Check sheet for the drawn part. Datum: minimum x, y, z corner. Units: mm. Coordinates: 2 decimals unless noted, no trailing zeros. Loops run counter-clockwise (first coordinate to the right, second up) from the corner with the lowest first, then second, coordinate; pieces in that order, holes last.
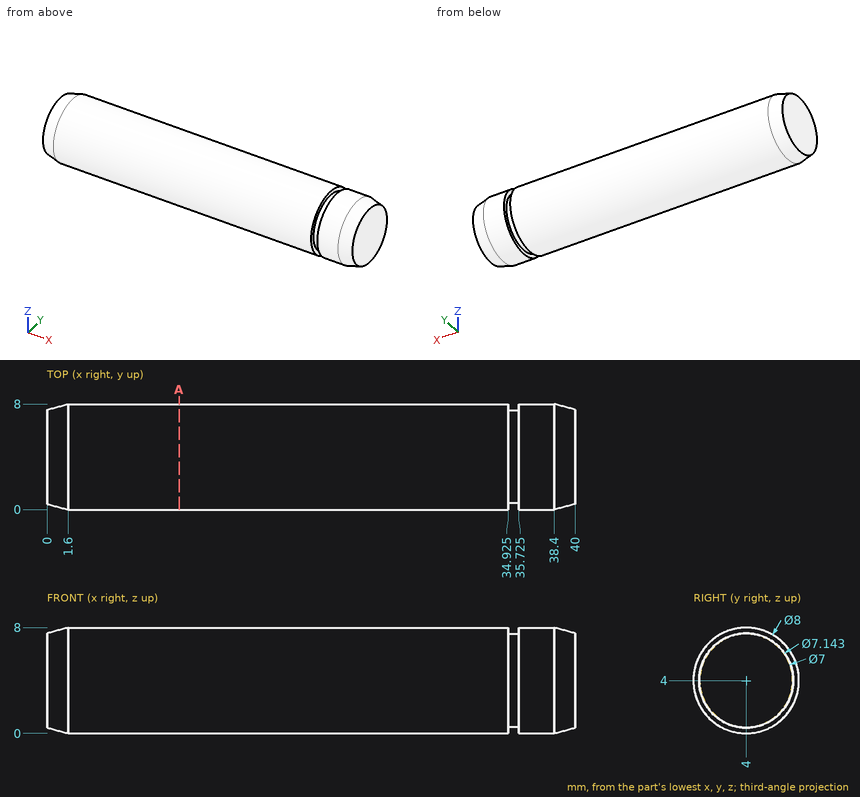
1) Section check A-A on x = 10. Enter the section's corners in (y, z).
Answer sheet:
outline: circle Ø8 at (4, 4)
2) Scan lines: line 1 (X direction, y = 3.5, z = 7.5) (1 decimal); line 2 (Y direction, x = 15, z = 3.75); line 3 (Y direction, x = 37, z = 0.5) (1 decimal). Record each from-to range of solid material in increasing order.
Answer sheet:
line 1: x = 0 to 34.9, 35.7 to 40
line 2: y = 0.01 to 7.99
line 3: y = 2.1 to 5.9
3) Depth check by flat-ended pin: pin 1 (1.5 mm diameter, centred on x = 7, z = 3, fed in from +Y); pin 2 (2 mm diameter, centred on x = 9, z = 7, fed in from +Y) (1 decimal); pin 3 (1 mm diameter, centred on x = 13, y = 6, fed in from +Z). Enter the tip coordinate at first touch or a pass-through.
Answer sheet:
pin 1: stops at y = 7.99
pin 2: stops at y = 7.5
pin 3: stops at z = 7.71
